Geometry: final body of the model. Coordinates: model frame, mm. A direction names the side the tool comes from. Round coordinates to 2 decimals unless told otherwise and drop trailing zeros. Order: outer loops, then holes, each group sorted by start corner. A loop starts at its lowest first (then second) coordinate and runs counter-clockwise, first axis right, second up. Notation, with made-up numbers: M 32.25,24 L 50.25,24 A19 cw 50.25,45 Z; hole C 50,69 d9. An arc over 180 degrees is marked long. Return JSON: item names as keys, results as strings. Group by question number.
Q1. Ray query, probe 1 along X at (y, z) = (1.85, 23.9); probe 2 along Z at (x, y) = (-37, 4); probe 3 along Z at (x, y) = (4.5, 3.5). Return the intervals inside material, ascending.
Q2. Contact query for flat-ended pins moving along their axis: pin 1 (3 mm diameter, centred on x = -27, z = -63, fed in from -Y); pin 2 (5 mm diameter, centred on x = 28.5, z = -55, fed in from +Y); pin 3 (0.5 mm diameter, centred on x = -12, y = 2.5, fed in from -Z); pin 4 (2 mm diameter, centred on x = -9.1, z = -9, fed in from +Y). Output: stop coordinate, or through.
Q3. Cut plane B-B on x = -15.5. Output: boundary loops of the cut face in (y, z), and give its area (3 significant figures).
Q4. Mould query, pull axis Z, two halves, no side actions, for faces 1 (the face through (-1, 3, 28)), 2 (the face through (-0.68, 5.366, 75.797)), 3 (the face through (47.5, 1, 1)). Classes: released by +Z, released by -Z, zero draft, split by the parting line, or undercut.
Q5. Cut plane A-A on x = 36. Output: boundary loops of the cut face in (y, z).
Q6. Access query for faces 4 (the face through (-1, 5, -17)), 5 (the face through (-45.3, 5, -1)), 6 (the face through (30.25, 2.86, -60.26)). Directions: +Z, -Z, +X, -X, +Y, -Y. A direction counts if a zero-diameter tool reaches every point of the face in a straight line with its end or side. Return the directions, or none.
```python
from build123d import *

# Parameters (mm, degrees)
SKETCH_1_R               = 1.65
EXTRUDE_1_DEPTH          = 3
SKETCH_2_R               = 1.65
EXTRUDE_2_DEPTH          = 4.8
SKETCH_7_R               = 3.5
SKETCH_7_R_2             = 1.65
CUT_EXTRUDE_1_DEPTH      = 4
SKETCH_8_R               = 3.25
CUT_EXTRUDE_2_DEPTH      = 5.8
SKETCH_9_W               = 86.6
SKETCH_9_H               = 3
EXTRUDE_3_DEPTH          = 4.8
SKETCH_11_R              = 1.15
CUT_EXTRUDE_3_DEPTH      = 8.8
CUT_EXTRUDE_4_DEPTH      = 5.8
CUT_EXTRUDE_4_DEPTH_BACK = 1


with BuildPart() as part:
    # 草图1 → 凸台-拉伸1 (new body)
    with BuildSketch(Plane(origin=(0, 0, 0), x_dir=(1, 0, 0), z_dir=(0, 1, 0))):
        with BuildLine():
            Line((-47.5, 61.868812822), (-47.5, -61.868812822))
            ThreePointArc((-47.5, -61.868812822), (0, -78), (47.5, -61.868812822))
            Line((47.5, -61.868812822), (47.5, 61.868812822))
            ThreePointArc((47.5, 61.868812822), (0, 78), (-47.5, 61.868812822))
        make_face()
        with Locations((-28.5, 63)):
            Circle(SKETCH_1_R, mode=Mode.SUBTRACT)
        with Locations((28.5, 63)):
            Circle(SKETCH_1_R, mode=Mode.SUBTRACT)
        with Locations((28.5, -63)):
            Circle(SKETCH_1_R, mode=Mode.SUBTRACT)
        with Locations((-28.5, -63)):
            Circle(SKETCH_1_R, mode=Mode.SUBTRACT)
    extrude(amount=EXTRUDE_1_DEPTH)

    # 草图2 → 凸台-拉伸2 (add)
    with BuildSketch(Plane(origin=(0, 3, 0), x_dir=(1, 0, 0), z_dir=(0, 1, 0))):
        with BuildLine():
            Line((-45.3, 60.774583503), (-45.3, -60.774583503))
            ThreePointArc((-45.3, -60.774583503), (0, -75.8), (45.3, -60.774583503))
            Line((45.3, -60.774583503), (45.3, 60.774583503))
            ThreePointArc((45.3, 60.774583503), (0, 75.8), (-45.3, 60.774583503))
        make_face()
        with Locations((-28.5, -63)):
            Circle(SKETCH_2_R, mode=Mode.SUBTRACT)
        with Locations((28.5, -63)):
            Circle(SKETCH_2_R, mode=Mode.SUBTRACT)
        with Locations((28.5, 63)):
            Circle(SKETCH_2_R, mode=Mode.SUBTRACT)
        with Locations((-28.5, 63)):
            Circle(SKETCH_2_R, mode=Mode.SUBTRACT)
        with BuildLine():
            Line((-43.3, 59.762446402), (-43.3, -59.762446402))
            ThreePointArc((-43.3, -59.762446402), (-37.862237267, -63.347383443), (-32.129574495, -66.438922649))
            ThreePointArc((-32.129574495, -66.438922649), (-26.439160651, -58.444460386), (-28.686460015, -67.996522057))
            ThreePointArc((-28.686460015, -67.996522057), (0, -73.8), (28.686460015, -67.996522057))
            ThreePointArc((28.686460015, -67.996522057), (26.439160651, -58.444460386), (32.129574495, -66.438922649))
            ThreePointArc((32.129574495, -66.438922649), (37.862237267, -63.347383443), (43.3, -59.762446402))
            Line((43.3, -59.762446402), (43.3, 59.762446402))
            ThreePointArc((43.3, 59.762446402), (37.862237267, 63.347383443), (32.129574495, 66.438922649))
            ThreePointArc((32.129574495, 66.438922649), (26.439160651, 58.444460386), (28.686460015, 67.996522057))
            ThreePointArc((28.686460015, 67.996522057), (0, 73.8), (-28.686460015, 67.996522057))
            ThreePointArc((-28.686460015, 67.996522057), (-26.439160651, 58.444460386), (-32.129574495, 66.438922649))
            ThreePointArc((-32.129574495, 66.438922649), (-37.862237267, 63.347383443), (-43.3, 59.762446402))
        make_face(mode=Mode.SUBTRACT)
    extrude(amount=EXTRUDE_2_DEPTH)

    # 草图7 → 切除-拉伸1 (cut, through all)
    with BuildSketch(Plane(origin=(0, 3, 0), x_dir=(1, 0, 0), z_dir=(0, 1, 0))):
        Circle(SKETCH_7_R)
        with Locations((9.1, 9)):
            Circle(SKETCH_7_R_2)
        with Locations((-9.1, 9)):
            Circle(SKETCH_7_R_2)
        with Locations((-9.1, -23.9)):
            Circle(SKETCH_7_R_2)
        with Locations((9.1, -23.9)):
            Circle(SKETCH_7_R_2)
    extrude(amount=-CUT_EXTRUDE_1_DEPTH, mode=Mode.SUBTRACT)

    # 草图8 → 切除-拉伸2 (cut)
    with BuildSketch(Plane.XZ):
        with Locations((-28.5, -63)):
            Circle(SKETCH_8_R)
        with Locations((28.5, -63)):
            Circle(SKETCH_8_R)
        with Locations((28.5, 63)):
            Circle(SKETCH_8_R)
        with Locations((-28.5, 63)):
            Circle(SKETCH_8_R)
    extrude(amount=-CUT_EXTRUDE_2_DEPTH, mode=Mode.SUBTRACT)

    # 草图9 → 凸台-拉伸3 (add)
    with BuildSketch(Plane(origin=(0, 3, 0), x_dir=(1, 0, 0), z_dir=(0, 1, 0))):
        with Locations((0, 18.5)):
            Rectangle(SKETCH_9_W, SKETCH_9_H)
    extrude(amount=EXTRUDE_3_DEPTH)

    # 草图11 → 切除-拉伸3 (cut, through all)
    with BuildSketch(Plane.XZ):
        with Locations((-8, -22)):
            Circle(SKETCH_11_R)
        with Locations((-11.249191362, -30.927079897)):
            Circle(SKETCH_11_R)
        with Locations((11.249191362, -30.927079897)):
            Circle(SKETCH_11_R)
        with Locations((8, -22)):
            Circle(SKETCH_11_R)
    extrude(amount=-CUT_EXTRUDE_3_DEPTH, mode=Mode.SUBTRACT)

    # 草图12 → 切除-拉伸4 (cut, two sides)
    with BuildSketch(Plane(origin=(0, 3, 0), x_dir=(1, 0, 0), z_dir=(0, 1, 0))) as cut_extrude_4_sk:
        Polygon((-10.06562331, 32.977079897), (-12.432759413, 32.977079897), (-13.616327465, 30.927079897), (-12.432759413, 28.877079897), (-10.06562331, 28.877079897), (-8.882055258, 30.927079897), align=None)
        Polygon((-5.632863896, 22), (-6.816431948, 24.05), (-9.183568052, 24.05), (-10.367136104, 22), (-9.183568052, 19.95), (-6.816431948, 19.95), align=None)
        Polygon((10.367136104, 22), (9.183568052, 24.05), (6.816431948, 24.05), (5.632863896, 22), (6.816431948, 19.95), (9.183568052, 19.95), align=None)
        Polygon((12.432759413, 32.977079897), (10.06562331, 32.977079897), (8.882055258, 30.927079897), (10.06562331, 28.877079897), (12.432759413, 28.877079897), (13.616327465, 30.927079897), align=None)
    extrude(amount=CUT_EXTRUDE_4_DEPTH, mode=Mode.SUBTRACT)
    extrude(cut_extrude_4_sk.sketch, amount=-CUT_EXTRUDE_4_DEPTH_BACK, mode=Mode.SUBTRACT)


solid = part.part
```
Result sheet:
{
 "1": {"probe 1": "x = -47.5 to -10.75, -7.45 to 7.45, 10.75 to 47.5", "probe 2": "z = -66.16 to -63.85, -20 to -17, 63.85 to 66.16", "probe 3": "z = -75.67 to -73.66, -20 to -17, 73.66 to 75.67"},
 "2": {"pin 1": "stops at y = 5.8", "pin 2": "stops at y = 3", "pin 3": "stops at z = -77.11", "pin 4": "passes through"},
 "3": {"outline": "M 0,-76.44 L 3,-76.44 L 3,-74.2 L 7.8,-74.2 L 7.8,-72.15 L 3,-72.15 L 3,-20 L 7.8,-20 L 7.8,-17 L 3,-17 L 3,72.15 L 7.8,72.15 L 7.8,74.2 L 3,74.2 L 3,76.44 L 0,76.44 Z", "area": "493 mm²"},
 "4": {"face 1": "undercut", "face 2": "released by +Z", "face 3": "zero draft"},
 "5": {"outline": "M 0,-69.2 L 3,-69.2 L 3,-66.71 L 7.8,-66.71 L 7.8,-64.42 L 3,-64.42 L 3,-20 L 7.8,-20 L 7.8,-17 L 3,-17 L 3,64.42 L 7.8,64.42 L 7.8,66.71 L 3,66.71 L 3,69.2 L 0,69.2 Z"},
 "6": {"face 4": "+Y", "face 5": "+Z, -Z, -X, +Y", "face 6": "-Y"}
}
